```python
from build123d import *

# Parameters (mm, degrees)
F1_R     = 2
F2_DEPTH = 3


with BuildPart() as f2:
    # F1 (on face) → F2 (new body)
    with BuildSketch(Plane.YZ):
        with BuildLine():
            Line((7.315274, 53.376805), (7.315274, 93.376805))
            ThreePointArc((7.315274, 93.376805), (-1.634726, 102.326805), (-10.584726, 93.376805))
            Line((-10.584726, 93.376805), (-10.584726, 53.376805))
            Line((-10.584726, 53.376805), (-30.584726, -41.623195))
            Line((-30.584726, -41.623195), (-16.584726, -41.623195))
            Line((-16.584726, -41.623195), (-8.723256, -0.514457))
            Line((-8.723256, -0.514457), (-8.95, 6.05))
            ThreePointArc((-8.95, 6.05), (-0.817363, 11.086847), (7.315274, 6.05))
            Line((7.315274, 6.05), (7.315274, -0.514457))
            Line((7.315274, -0.514457), (13.315274, -41.623195))
            Line((13.315274, -41.623195), (27.315274, -41.623195))
            Line((27.315274, -41.623195), (7.315274, 53.376805))
        make_face()
        with Locations((-1.634726, 93.376805)):
            Circle(F1_R, mode=Mode.SUBTRACT)
    extrude(amount=F2_DEPTH)


solid = f2.part
```
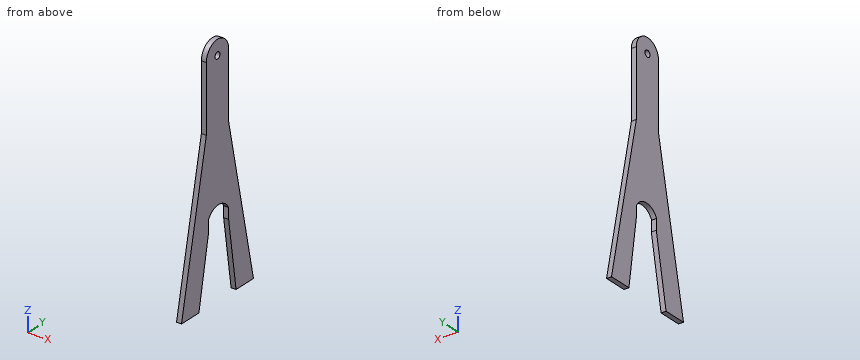
The listing builds one solid part. Answer for the finished solid, in the listing's coordinates (mm). Coordinates: 2 decimals unless noted, no trailing zeros. Write each loop counter-clockwise with the first axis right and the second up, starting at its lowest first coordinate (ties: lowest second). Pieces come first, ordered by that corner, then holes. Notation, with made-up numbers: (32.25, 3.25) - (87.25, 3.25) arc R29 cw to (87.25, 42.25) - close; hole circle Ø4 at (64.25, 20). An arc over 180 degrees is marked (long way). Return JSON: item names as keys, results as strings. Group by question number.
1. Given pin 1 (1.5 mm diameter, centred on x = 2, z = 41, fed in from -Y); pin 2 (0.9 mm diameter, centred on x = 1.5, z = 79, fed in from +Y); pin 3 (12 mm diameter, centred on y = -17, z = 58.5, fed in from +X), each flat-ended and moving along its own axis, determine where each tip first touches the part or whether it passes through.
2. A cutting plane is placed at D-D, the plane z = 78.5. Determine the outline of the cut face in (x, y), plus the area to 3 significant figures.
3. A cutting plane is placed at C-C, the plane x = 2.2. Determine the outline of the cut face in (y, z).
4. Straight lines are drawn through the part: L1, parallel to Y at x = 1.8, z = -22.5; L2, parallel to Z at x = 2.6, y = -3; L3, parallel to Y at x = 2.6, z = -4. For each, find the intervals that lie inside material, in ascending order.
5. A cutting plane is placed at B-B, the plane y = -2. Determine the outline of the cut face in (x, z), plus the area to 3 significant figures.
6. A cutting plane is placed at A-A, the plane z = -26. Determine the outline of the cut face in (x, y) (3 decimals).
Ans:
{
 "1": {"pin 1": "y = -13.35", "pin 2": "y = 7.32", "pin 3": "through"},
 "2": {"outline": "(0, -10.58) - (3, -10.58) - (3, 7.32) - (0, 7.32) - close", "area": "53.7 mm²"},
 "3": {"outline": "(-30.58, -41.62) - (-16.58, -41.62) - (-8.72, -0.51) - (-8.95, 6.05) arc R9.08 cw to (7.32, 6.05) - (7.32, -0.51) - (13.32, -41.62) - (27.32, -41.62) - (7.32, 53.38) - (7.32, 93.38) arc R8.95 ccw to (-10.58, 93.38) - (-10.58, 53.38) - close; hole circle Ø4 at (-1.63, 93.38)"},
 "4": {"L1": "-26.56 to -12.93, 10.52 to 23.29", "L2": "10.82 to 91.92, 94.84 to 102.22", "L3": "-22.66 to -9.39, 7.82 to 19.39"},
 "5": {"outline": "(0, 11.01) - (3, 11.01) - (3, 91.41) - (0, 91.41) - close; (0, 95.34) - (3, 95.34) - (3, 102.32) - (0, 102.32) - close", "area": "262 mm²"},
 "6": {"outline": "(0, -27.296) - (3, -27.296) - (3, -13.597) - (0, -13.597) - close; (0, 11.035) - (3, 11.035) - (3, 24.026) - (0, 24.026) - close"}
}
